Autodesk Inventor part; units mm, degrees
ref_plane "Work Plane1" through (30, -47.6627, 1.8405) normal (-1, 0, 0) x (0, -0.3826834, 0.9238795)
ref_plane "Work Plane2" through (-30, -31.4, -6.35) normal (0, -1, 0) x (1, 0, 0)
ref_plane "YZ Plane" through (0, 0, 0) normal (1, 0, 0) x (0, 1, 0)
sketch "Sketch1" plane through (0, 0, 0) normal (0, 0, 1) x (1, 0, 0)
  circle A0 centre (20, -21.4) radius 2.5
  circle A1 centre (20, 21.4) radius 2.5
  circle A2 centre (-20, -21.4) radius 2.5
  circle A3 centre (-20, 21.4) radius 2.5
  line L0 (-30, 31.4) -> (-30, -31.4)
  line L1 (-30, -31.4) -> (30, -31.4)
  line L2 (30, -31.4) -> (30, 31.4)
  line L3 (30, 31.4) -> (-30, 31.4)
  line L4 (-30, -44.5) -> (60, -44.5)
  line L5 (60, -44.5) -> (60, -30.5)
  line L6 (-30, -30.5) -> (60, -30.5)
  line L7 (-30, -31.4) -> (30, -31.4)
  line L8 (30, -31.4) -> (30, -11.4)
  line L9 (30, -11.4) -> (-30, -11.4)
  line L10 (-30, -11.4) -> (-30, -31.4)
  line L11 (30, -11.4) -> (-30, -11.4)
  line L12 (-30, -11.4) -> (-30, -28.7084)
  line L13 (-30, -28.7084) -> (30, -28.7084)
  line L14 (30, -28.7084) -> (30, -11.4)
  point P0 (0, 0)
  dimension "d0" = 20
  dimension "d1" = 0
extrude "Extrusion1" add sketch "Sketch1" along normal blind 4 contours L9 L2 L13 L0
ref_plane "Work Plane1" through (30, -47.6627, 1.8405) normal (-1, 0, 0) x (0, -0.3826834, 0.9238795)
sketch "Sketch2" plane through (30, -47.6627, 1.8405) normal (-1, 0, 0) x (0, -0.3826834, 0.9238795)
  circle A0 centre (0, 11) radius 4
  arc A1 (-10.7913, 13.1327) -> (-9.1051, 17.1723) centre (0, 11) ccw
  line L0 (-5.2583, 18.3379) -> (-11.882, 34.3288)
  line L1 (-5.9532, -3.3722) -> (-10.1627, 6.7905)
  line L2 (5.9532, 25.3722) -> (14.3722, 5.0468)
  line L3 (14.3722, 5.0468) -> (-5.9532, -3.3722)
  line L4 (-5.9532, -3.3722) -> (5.9532, 25.3722) construction
  line L5 (-14.3722, 16.9532) -> (14.3722, 5.0468) construction
  line L6 (-7.9238, 14.3204) -> (-13.7905, 11.8904)
  line L7 (-7.9238, 14.3204) -> (-31.9564, 72.3401)
  line L8 (-4.2095, 21.1627) -> (5.9532, 25.3722)
  line L9 (-28.0775, 29.1357) -> (1.083, -41.2639)
  circle A2 centre (7.391, 14.0615) radius 1.5
  circle A3 centre (-7.391, 7.9385) radius 1.5
  circle A4 centre (-3.0615, 18.391) radius 1.5
  circle A5 centre (3.0615, 3.609) radius 1.5
  circle A6 centre (0, 11) radius 4
  circle A7 centre (0, 11) radius 11
  point P0 (-19.9401, 43.3302)
extrude "Extrusion2" add sketch "Sketch2" along normal blind 4 contours L6 L7 A1 | A1 L3 L1 | A1 L2 L3 | L8 L2 A1
sketch "Sketch3" plane through (30, -11.4, 4) normal (1, 0, 0) x (0, 0, -1)
  line L0 (-13.05, -15.1) -> (-2.05, -15.1)
  line L1 (-13.05, -15.1) -> (0, 0)
  arc A0 (0, -15.2927) -> (-2.05, -15.1) centre (-2.05, -26.1) ccw
  line L2 (0, 0) -> (0, -15.2927)
  line L3 (0, -15.2927) -> (-13.05, -15.1)
  point P0 (4, 11.4)
extrude "Extrusion3" add sketch "Sketch3" against normal up to surface (4 mm away) contours L1 L2 A0 L0
sketch "Sketch6" plane through (26, -47.6627, 1.8405) normal (-1, 0, 0) x (0, -0.3826834, 0.9238795)
  circle A0 centre (-3.0615, 18.391) radius 1.5
  circle A1 centre (-3.0615, 18.391) radius 2.75
  point P0 (-19.9401, 43.3302)
  dimension "d10" = 5.5
extrude "Extrusion5" add sketch "Sketch6" against normal up to surface (4 mm away) contours A0
sketch "Sketch7" plane through (-30, -28.7084, 0) normal (0, -1, 0) x (1, 0, 0)
  line L0 (56, 17.05) -> (42.95, 4)
  line L1 (0, 4) -> (56, 4)
  line L2 (42.95, 4) -> (56, 4)
  line L3 (56, -4.95) -> (56, 17.05)
  line L4 (56, 4) -> (56, 17.05)
  point P0 (30, 0)
  dimension "d13" = 45
extrude "Extrusion6" add sketch "Sketch7" against normal up to surface (2.2084 mm away)
sketch "Sketch8" plane through (-30, -28.7084, 0) normal (0, -1, 0) x (1, 0, 0)
  line L0 (56, 0) -> (56, 17.05)
  line L1 (56, 17.05) -> (42.95, 4)
  line L2 (0, 4) -> (42.95, 4)
  line L3 (0, 0) -> (0, 4)
  line L4 (0, 0) -> (56, 0)
  line L5 (0, 0) -> (56, 0)
  line L6 (0, 0) -> (56, 0)
  line L7 (56, 0) -> (56, 4)
  line L8 (56, 4) -> (0, 4)
  line L9 (0, 4) -> (0, 0)
  point P0 (30, 0)
ref_plane "Work Plane2" through (-30, -31.4, -6.35) normal (0, -1, 0) x (1, 0, 0)
extrude "Extrusion7" add sketch "Sketch8" along normal up to surface (2.6916 mm away) contours L4 L3 L2 L8 L0
sketch "Sketch10" plane through (12.95, -28.7084, 4) normal (0, -1, 0) x (1, 0, 0)
  line L0 (0, 0) -> (13.05, 0)
  line L1 (13.05, 0) -> (13.05, 13.05)
  line L2 (13.05, 13.05) -> (0, 0)
  point P0 (-12.95, -4)
extrude "Extrusion8" add sketch "Sketch10" along normal up to surface (2.6916 mm away)
sketch "Sketch12" plane through (26, -47.6627, 1.8405) normal (-1, 0, 0) x (0, -0.3826834, 0.9238795)
  circle A0 centre (7.391, 14.0615) radius 1.5
  circle A1 centre (-7.391, 7.9385) radius 1.5
  circle A2 centre (3.0615, 3.609) radius 1.5
  circle A3 centre (0, 11) radius 4
  line L0 (7.8283, 20.8452) -> (-7.9238, 14.3204)
  line L1 (-7.9238, 14.3204) -> (-10.7913, 13.1327)
  arc A4 (-10.7913, 13.1327) -> (-10.1627, 6.7905) centre (0, 11) ccw
  line L2 (-10.1627, 6.7905) -> (-5.9532, -3.3722)
  line L3 (-5.9532, -3.3722) -> (14.3722, 5.0468)
  line L4 (14.3722, 5.0468) -> (7.8283, 20.8452)
  line L5 (-10.1627, 6.7905) -> (-12.497, 12.4261)
  line L6 (-10.1627, 6.7905) -> (-5.9532, -3.3722)
  line L7 (-10.7913, 13.1327) -> (-12.497, 12.4261)
  line L8 (-7.9238, 14.3204) -> (-10.7913, 13.1327)
  point P0 (-19.9401, 43.3302)
extrude "Extrusion9" add sketch "Sketch12" against normal up to surface (4 mm away) contours A4 L5 L7
fillet "Fillet1" radius 11 2 edges at (28, -48.5, 17.05) (28, -48.5, -4.95)
sketch "Sketch15" plane through (30, -31.4, 0) normal (1, 0, 0) x (0, 0, -1)
  circle A0 centre (-6.05, -6.1) radius 4
  circle A1 centre (-6.05, -6.1) radius 5.27
  point P0 (0, 31.4)
  dimension "d24" = 1.27
extrude "Extrusion10" cut sketch "Sketch15" against normal through all
properties part number "nutHolderX"
The listing builds one solid part. Answer for the finished solid, in the listing's coordinates (mm). A direction names the side the tool comes from. Give positions to 0.01 mm unless a question says otherwise; leave off trailing zeros. Order: outer loops, then holes, each group sorted by start corner. A loop starts at its lowest first (then second) coordinate and runs counter-clockwise, first axis right, second up. Notation, with made-up numbers: (87, -5.5) -> (127, -5.5) arc R22 ccw to (127, 20.5) -> close; hole circle Ø7 at (45, 60). An arc over 180 degrees is marked (long way). Answer as CSV lines item,"result". Start each with the question number.
Q1. A cutting plane is placed at D-D (x = 20). Determine the outline of the cut face in (y, z), then the cut area to 3 significant figures.
Q2. Given pin 1 (4 mm diameter, centred on y = -37.5, z = 14.05, fed in from -X); pin 2 (1.6 mm diameter, centred on x = 27, z = -2.5, fed in from +Y); pin 3 (8 mm diameter, centred on x = -2, y = -36.5, fed in from -Z); pin 4 (2 mm diameter, centred on x = 28, y = -29.5, fed in from -Z), each flat-ended and moving along its own axis, determine where each tip first touches the part or whether it passes through.
Q3. A cutting plane is placed at C-C (y = -41.5). Determine the outline of the cut face in (x, z).
Q4. Which of the six approach directions +Z, -Z, +X, -X, +Y, -Y give full straight-line access (tool end or side, diameter ignored) to faces 5 (the cylindrical face through (28.028, -32.275, 6.736)), 6 (the flat face through (22, -26.5, 8)), 7 (the flat face through (4, -31.4, 2))?
Q5. Find the intervals of material crossed by L1, parallel to X at y = -24.5, z = 5.5; L2, parallel to Y at x = 16.5, z = 6; L3, parallel to Y at x = 20, z = 1.6, in increasing order.
Q6. A cutting plane is placed at B-B (y = -21.4). Determine the outline of the cut face in (x, z), then the cut area to 3 significant figures.
Q7. A cutting plane is placed at A-A (x = -20). Determine the outline of the cut face in (y, z).
Q8. Determine the mould class of faces 1 (the flat face through (19.57, -28.92, 10.62)), 2 (the cylindrical face through (27.972, -45.363, 13.742)), 3 (the cylindrical face through (-21.84, -23.09, 1.97)), 4 (the flat face through (0, -11.4, 2)) for opening direction Y: pulls with the +Y half, pulls with the -Y half, needs draft (parallel to the pull), parting line crosses it, or undercut.
Results found:
1,outline,"(-31.4, 0) -> (-23.9, 0) -> (-23.9, 4) -> (-26.5, 4) -> (-26.5, 11.05) -> (-31.4, 11.05) -> close; (-18.9, 0) -> (-11.4, 0) -> (-11.4, 4) -> (-18.9, 4) -> close"
1,area,"94.5 mm2"
2,pin 1,"x = 26"
2,pin 2,"y = -31.4"
2,pin 3,"through"
2,pin 4,"z = 0"
3,outline,"(26, -4.2) -> (30, -4.2) -> (30, 2.62) -> (26, 2.62) -> close; (26, 9.48) -> (30, 9.48) -> (30, 16.3) -> (26, 16.3) -> close"
4,face 5,"+X, -X"
4,face 6,"+Z, -X, +Y"
4,face 7,"+Z, -Z, -X, -Y"
5,L1,"26 to 30"
5,L2,"-31.4 to -26.5"
5,L3,"-31.4 to -23.9, -18.9 to -11.4"
6,outline,"(-30, 0) -> (-22.5, 0) -> (-22.5, 4) -> (-30, 4) -> close; (-17.5, 0) -> (17.5, 0) -> (17.5, 4) -> (-17.5, 4) -> close; (22.5, 0) -> (30, 0) -> (30, 12.64) -> (26, 12.64) -> (26, 4) -> (22.5, 4) -> close"
6,area,"235 mm2"
7,outline,"(-31.4, 0) -> (-23.9, 0) -> (-23.9, 4) -> (-31.4, 4) -> close; (-18.9, 0) -> (-11.4, 0) -> (-11.4, 4) -> (-18.9, 4) -> close"
8,face 1,"needs draft"
8,face 2,"pulls with the -Y half"
8,face 3,"undercut"
8,face 4,"pulls with the +Y half"
